```python
from build123d import *

# Parameters (mm, degrees)
BOSS_EXTRUDE1_DEPTH = 7.25
BOSS_EXTRUDE2_START = -1.75
BOSS_EXTRUDE2_DEPTH = 0.5
CHAMFER1_SIZE       = 0.2


with BuildPart() as part:
    # Sketch1 → Boss-Extrude1 (new, symmetric)
    with BuildSketch(Plane(origin=(0, 0, 0), x_dir=(1, 0, 0), z_dir=(0, 1, 0))):
        with BuildLine():
            Line((-1.25, -3), (1.25, -3))
            ThreePointArc((1.25, -3), (0, 3.25), (-1.25, -3))
        make_face()
    extrude(amount=BOSS_EXTRUDE1_DEPTH, both=True)

    # Sketch2 → Boss-Extrude2 (add)
    with BuildSketch(Plane.XZ.offset(7.25).offset(BOSS_EXTRUDE2_START)):
        with BuildLine():
            Line((-1.25, 3), (-1.6, 3))
            ThreePointArc((-1.6, 3), (0, -3.4), (1.6, 3))
            Line((1.6, 3), (1.25, 3))
            ThreePointArc((1.25, 3), (0, -3.25), (-1.25, 3))
        make_face()
    extrude(amount=BOSS_EXTRUDE2_DEPTH)

    # Chamfer1
    # the kernel refuses this chamfer: 0.2 mm, written as the material it takes off along each edge
    with BuildSketch(Plane(origin=(0, -5.5, 0), x_dir=(-0.3315887986155938, 0, 0.9434240131736458), z_dir=(0.9434240131736458, 0, 0.3315887986155938))) as chamfer1_piece_1_section:
        Polygon((3.4, CHAMFER1_SIZE), (3.4 - CHAMFER1_SIZE, 0), (3.4, 0), align=None)
    chamfer1_piece_1 = revolve(axis=Axis((0, -5.5, 0), (0, -1, 0)), revolution_arc=321.269525005, mode=Mode.PRIVATE)
    chamfer1_piece_1 = chamfer1_piece_1 - Plane(origin=(0, -5.5, 0), x_dir=(0.38461538461538497, 0, 0.923076923076923), z_dir=(0, 1, 0)) * Cylinder(3.25, 14, mode=Mode.PRIVATE)
    add(chamfer1_piece_1, mode=Mode.SUBTRACT)

    # Chamfer2: read off the stored shape, not the designer's step
    # Chamfer2 outline → Chamfer2 (revolve, cut)
    with BuildSketch(Plane.XY):
        Polygon((3.25, 7.25), (2.75, 7.25), (3.25, 6.75), align=None)
    revolve(axis=Axis((0, 0, 0), (0, 1, 0)), mode=Mode.SUBTRACT)


solid = part.part
```
Read the model definition and answer for the solid it produces. Units are mm, in the model's axes. A direction names the side the tool comes from. Coordinates: 2 decimals unless noted, no trailing zeros. Write each loop counter-clockwise with the first axis right and the second up, starting at its lowest first coordinate (ties: lowest second). Pieces come first, ordered by that corner, then holes. Notation, with made-up numbers: (62, 43.25) -> (86, 43.25) arc R24 cw to (86, 62.25) -> close; hole circle Ø9 at (-12.75, 43). An arc over 180 degrees is marked (long way). Answer as a JSON object with one key per item and string values.
Q1. Flat-ended cylindrical pins translate along their axes: pin 1 Ø2 at (y, z) = (4.5, 0.5) entering from -X; pin 2 Ø4 at (x, y) = (-0.5, -2) entering from -Z. Find the tip coordinate at first contact, or state that the pin passes through.
The answers:
{"pin 1": "stops at x = -3.25", "pin 2": "stops at z = -3.25"}
Q2. The part is cut by section C-C on y = -2. Give the vertices of the cut face in (x, z), then the cut area to 3 significant figures.
The answers:
{"outline": "(-1.25, 3) arc R3.25 ccw (long way) to (1.25, 3) -> close", "area": "32.8 mm2"}
Q3. Consider line 1 (Z direction, x = 0, y = 6.25); line 2 (Z direction, x = -2, y = -4); line 3 (Y direction, x = 0.5, z = -2.75). Determine where each line is inside the solid, lowest interval first. Write a range as [from, to].
The answers:
{"line 1": "z = [-3.25, 3]", "line 2": "z = [-2.56, 2.56]", "line 3": "y = [-7.25, 7.2]"}
Q4. The part is cut by section A-A on x = 0. Give the vertices of the cut face in (y, z).
The answers:
{"outline": "(-7.25, -3.25) -> (-6, -3.25) -> (-6, -3.4) -> (-5.7, -3.4) -> (-5.55, -3.25) -> (6.75, -3.25) -> (7.25, -2.75) -> (7.25, 2.75) -> (7, 3) -> (-7.25, 3) -> close"}
Q5. The part is cut by section B-B on z = 0. Give the vertices of the cut face in (x, y), then the cut area to 3 significant figures.
The answers:
{"outline": "(-3.4, -6) -> (-3.25, -6) -> (-3.25, -7.25) -> (3.25, -7.25) -> (3.25, -6) -> (3.4, -6) -> (3.4, -5.7) -> (3.25, -5.55) -> (3.25, 6.75) -> (2.75, 7.25) -> (-2.75, 7.25) -> (-3.25, 6.75) -> (-3.25, -5.55) -> (-3.4, -5.7) -> close", "area": "94.1 mm2"}
Q6. A tool of negligible diameter and unlimited length cuts with its end or side. For faces 1 (the cylindrical face through (0.125, 0.686, -3.248)), 2 (the cylindrical face through (0.125, -6.616, -3.248)), 3 (the flat face through (0, 0, 3)), from which of +Z, -Z, +X, -X, +Y, -Y can it reach the whole face along a straight path? Write none if from no direction.
The answers:
{"face 1": "+Y", "face 2": "-Y", "face 3": "+Z, +X, -X, +Y, -Y"}
